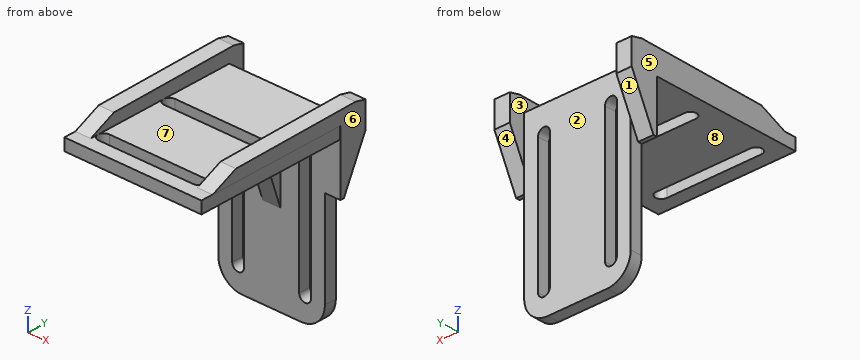
Autodesk Inventor part; units mm, degrees
ref_plane "XY Plane" through (0, 0, 0) normal (0, 0, 1) x (1, 0, 0)
sketch "Sketch1" plane through (0, 0, 0) normal (0, 1, 0) x (-1, 0, 0)
  line L0 (-9, 20) -> (9, 20)
  line L1 (9, 20) -> (9, -10.6569)
  line L2 (9, -10.6569) -> (-9, -10.6569)
  line L3 (-9, -10.6569) -> (-9, 20)
  line L4 (-9, 20) -> (9, -10.6569) construction
  line L5 (9, 20) -> (-9, -10.6569) construction
  line L6 (0, -28.0453) -> (0, 28.0076) construction
  line L7 (-14.8076, 0) -> (25.8453, 0) construction
  line L8 (0, 0) -> (20.0378, -20.0378) construction
  line L9 (5.6569, -7.6569) -> (5.6569, 16.6569) construction
  line L10 (6.6569, -6.6569) -> (6.6569, 15.6569)
  line L11 (4.6569, 15.6569) -> (4.6569, -6.6569)
  arc A0 (4.6569, -6.6569) -> (6.6569, -6.6569) centre (5.6569, -6.6569) ccw
  arc A1 (6.6569, 15.6569) -> (4.6569, 15.6569) centre (5.6569, 15.6569) ccw
  line L12 (0, 0) -> (13.8345, 13.8345) construction
  line L13 (-5.6569, -7.6569) -> (-5.6569, 16.6569) construction
  line L14 (-6.6569, -6.6569) -> (-6.6569, 15.6569)
  line L15 (-4.6569, 15.6569) -> (-4.6569, -6.6569)
  arc A2 (-6.6569, -6.6569) -> (-4.6569, -6.6569) centre (-5.6569, -6.6569) ccw
  arc A3 (-4.6569, 15.6569) -> (-6.6569, 15.6569) centre (-5.6569, 15.6569) ccw
  point P0 (0, 4.6716)
  point P1 (0, 4.6716)
  point P2 (5.6569, -5.6569)
  point P3 (5.6569, 4.5)
  point P4 (5.6569, 5.6569)
  point P5 (-5.6569, -5.6569)
  point P6 (-5.6569, 4.5)
  point P7 (-5.6569, 5.6569)
  dimension "d34" = 18
  dimension "d35" = 45
  dimension "d36" = 8
  dimension "d37" = 2
  dimension "d38" = 1
  dimension "d40" = 45
  dimension "d41" = 10
  dimension "d42" = 4
  dimension "d43" = 20
extrude "Extrusion1" add sketch "Sketch1" against normal blind 2
sketch "Sketch5" plane through (-9, 0, 20) normal (0, 0, 1) x (1, 0, 0)
  line L0 (-2.5982, 0) -> (20.5467, 0)
  line L1 (20.5467, 0) -> (20.5467, -27.3268)
  line L2 (20.5467, -27.3268) -> (-2.5982, -27.3268)
  line L3 (-2.5982, -27.3268) -> (-2.5982, 0)
  line L4 (18, 0) -> (18, -2) construction
  line L5 (0, 0) -> (0, -2)
  line L6 (1, -24) -> (17, -24) construction
  line L7 (1, -25) -> (17, -25)
  line L8 (17, -23) -> (1, -23)
  arc A0 (1, -23) -> (1, -25) centre (1, -24) ccw
  arc A1 (17, -25) -> (17, -23) centre (17, -24) ccw
  line L9 (1, -12) -> (17, -12) construction
  line L10 (1, -13) -> (17, -13)
  line L11 (17, -11) -> (1, -11)
  arc A2 (1, -11) -> (1, -13) centre (1, -12) ccw
  arc A3 (17, -13) -> (17, -11) centre (17, -12) ccw
  line L12 (0, -2) -> (18, -2)
  point P0 (9, 0)
  point P1 (9, -24)
  point P2 (9, -12)
  dimension "d56" = 2
  dimension "d57" = 2
  dimension "d58" = 12
  dimension "d59" = 8
  dimension "d62" = 10
extrude "Extrusion5" add sketch "Sketch5" against normal blind 2
ref_plane "Work Plane1" through (-8, -18, 20) normal (0, -1, 0) x (1, 0, 0)
fillet "Fillet2" radius 4 2 edges at (-9, -1, -10.6569) (9, -1, -10.6569)
sketch "Sketch6" plane through (0, 0, 0) normal (1, 0, 0) x (0, 1, 0)
  line L0 (-2, 4.2697) -> (-6.6287, 18)
  line L1 (-6.6287, 18) -> (-2, 18)
  line L2 (-2, 18) -> (-2, -6.6569)
  line L3 (-2, 18) -> (-2, 4.2697)
  point P0 (0, 0)
extrude "Extrusion6" add sketch "Sketch6" along normal mid plane 3
sketch "Sketch7" plane through (-9, -2, 18) normal (-1, 0, 0) x (0, 0, 1)
  line L0 (-8.6385, 0.6553) -> (-0.5065, 4.6311)
  line L1 (-0.5065, 4.6311) -> (3.8294, 4.6311)
  line L2 (3.8294, 4.6311) -> (4.27, 2.7989)
  line L3 (4.27, 2.7989) -> (3.937, -19.0711)
  line L4 (3.937, -19.0711) -> (2, -23.3264)
  line L5 (-8.6385, 0.6553) -> (-8.6385, 0)
  line L6 (2, 0) -> (2, -23.3264)
  line L7 (2, 0) -> (-8.6385, 0)
  line L8 (0, 0) -> (-24.6569, 0)
  point P0 (-18, 2)
  point P1 (2, 2)
extrude "Extrusion7" add sketch "Sketch7" along normal up to surface (2.5982 mm away)
mirror "Mirror1" about plane through (0, 0, 0) normal (1, 0, 0) of "Extrusion7"
properties part number "gimbal_pitch_brushless" material "ABS Plastic"
Can you work these out from the model? Positions are in its coordinate system, mm. Face numbers are marked on the shaded views. A direction names the side the tool comes from. Round coordinates to 2 decimals unless told otherwise and drop trailing zeros. Order: outer loops, then holes, each group sorted by start corner. A loop starts at its lowest first (then second) coordinate and runs counter-clockwise, first axis right, second up. Notation, with made-up numbers: (26, -24) -> (65, -24) arc R19 ccw to (65, 3) -> close; hole circle Ø8 at (-6.75, 36.5). An arc over 180 degrees is marked (long way). Write each question's results on one line, items separated by ' | '. Start each with the question number.
Item 1: Which directions (+Z, -Z, +X, -X, +Y, -Y) give clear straight access to the entire face, cutting with the end or side of a thin tool? Please do the marked faces 1, 2, 3 and 4.
Item 2: If we section it at A-A, the plane z = 2.5: Write out the boundary of the cut face in (x, y), then the cut area to 3 significant figures.
Item 3: Please list where these lines run through material, in increasing order: L1, parallel to X at y = -0.25, z = -1; L2, parallel to X at y = -5.25, z = 14; L3, parallel to Y at x = -1.75, z = 9.5.
Item 4: If we section it at B-B, the plane x = 3.5: Write out the boundary of the cut face in (y, z).
Item 5: Will these pins go through, and if not, where does the flat tip stop? pin 1 (0.7 mm diameter, centred on x = -10.5, y = -1.5, fed in from -Z); pin 2 (3 mm diameter, centred on x = 3.5, z = -2, fed in from -Y); pin 3 (9 mm diameter, centred on x = 0, z = 8.5, fed in from +Y); pin 4 (2 mm diameter, centred on y = -4.5, z = -5, fed in from -X).
Item 6: If we section it at C-C, the plane y = -0.75: Write out the boundary of the cut face in (x, z).
Item 7: If we section it at D-D, the plane z = 7.5: Write out the boundary of the cut face in (x, y).
Item 8: Thinking about a two-plate mould opening in X: for the marked faces 5, 6, 7 and 8, which applies, +X half, -X half, draft (parallel to the pull), parting line (faces both ways), or undercut?
Results:
1) face 1: -Z, -X, +Y | face 2: +Z, -Z, +Y | face 3: +Z, +Y | face 4: -Z, +X, +Y
2) outline: (-9, -2) -> (-6.66, -2) -> (-6.66, 0) -> (-9, 0) -> close; (-4.66, -2) -> (4.66, -2) -> (4.66, 0) -> (-4.66, 0) -> close; (6.66, -2) -> (9, -2) -> (9, 0) -> (6.66, 0) -> close | area: 28.0 mm2
3) L1: x = -9 to -6.66, -4.66 to 4.66, 6.66 to 9 | L2: x = -1.5 to 1.5 | L3: y = -2 to 0
4) outline: (-27.33, 18) -> (-25, 18) -> (-25, 20) -> (-27.33, 20) -> close; (-23, 18) -> (-13, 18) -> (-13, 20) -> (-23, 20) -> close; (-11, 18) -> (-2, 18) -> (-2, -10.66) -> (0, -10.66) -> (0, 20) -> (-11, 20) -> close
5) pin 1: stops at z = 9.36 | pin 2: stops at y = -2 | pin 3: stops at y = 0 | pin 4: passes through
6) outline: (-11.6, 10.58) -> (-9, 10.58) -> (-9, -6.66) arc R4 ccw to (-5, -10.66) -> (5, -10.66) arc R4 ccw to (9, -6.66) -> (9, 10.58) -> (11.6, 10.58) -> (11.6, 22.25) -> (9, 22.25) -> (9, 20) -> (-9, 20) -> (-9, 22.25) -> (-11.6, 22.25) -> close; hole (-6.66, -6.66) arc R1 ccw to (-4.66, -6.66) -> (-4.66, 15.66) arc R1 ccw to (-6.66, 15.66) -> close; hole (4.66, -6.66) arc R1 ccw to (6.66, -6.66) -> (6.66, 15.66) arc R1 ccw to (4.66, 15.66) -> close
7) outline: (-9, -2) -> (-6.66, -2) -> (-6.66, 0) -> (-9, 0) -> close; (-4.66, -2) -> (-1.5, -2) -> (-1.5, -3.09) -> (1.5, -3.09) -> (1.5, -2) -> (4.66, -2) -> (4.66, 0) -> (-4.66, 0) -> close; (6.66, -2) -> (9, -2) -> (9, 0) -> (6.66, 0) -> close
8) face 5: -X half | face 6: +X half | face 7: undercut | face 8: draft
